```python
from build123d import *
from build123d import SkipClean  # not in build123d's __all__

# Parameters (mm, degrees)
F0_R     = 2.032
F1_DEPTH = 4.7625
F2_W     = 10.16
F2_H     = 58.42
F3_DEPTH = 6.35


with BuildPart() as f1:
    # F0 (on Top) → F1 (new body, symmetric)
    with BuildSketch(Plane.XY):
        with BuildLine():
            Line((0, -37.2616276145), (0, -45.72))
            add(Edge.make_bspline(
                [(0, -45.72), (28.8508510644, -45.72), (44.8791016558, -25.4)],
                knots=[1.5707963268, 1.5707963268, 1.5707963268, 2.5525616834, 2.5525616834, 2.5525616834], degree=2, weights=[1, 0.8819171037, 1]))
            Line((44.8791016558, -25.4), (44.8791016558, -23.9395))
            Line((44.8791016558, -23.9395), (37.2591016558, -23.9395))
            Line((37.2591016558, -23.9395), (37.2591016558, -19.4183))
            Line((37.2591016558, -19.4183), (30.7821016558, -19.4183))
            Line((30.7821016558, -19.4183), (30.7821016558, -21.1963))
            Line((30.7821016558, -21.1963), (26.7181016558, -21.1963))
            Line((26.7181016558, -21.1963), (26.7181016558, -13.5763))
            Line((26.7181016558, -13.5763), (30.7821016558, -13.5763))
            Line((30.7821016558, -13.5763), (30.7821016558, -15.3543))
            Line((30.7821016558, -15.3543), (37.2591016558, -15.3543))
            Line((37.2591016558, -15.3543), (37.2591016558, 15.2273))
            Line((37.2591016558, 15.2273), (30.7821016558, 15.2273))
            Line((30.7821016558, 15.2273), (30.7821016558, 13.4493))
            Line((30.7821016558, 13.4493), (26.7181016558, 13.4493))
            Line((26.7181016558, 13.4493), (26.7181016558, 21.0693))
            Line((26.7181016558, 21.0693), (30.7821016558, 21.0693))
            Line((30.7821016558, 21.0693), (30.7821016558, 19.2913))
            Line((30.7821016558, 19.2913), (37.2591016558, 19.2913))
            Line((37.2591016558, 19.2913), (37.2591016558, 23.8125))
            Line((37.2591016558, 23.8125), (44.8791016558, 23.8125))
            Line((44.8791016558, 23.8125), (44.8791016558, 25.4))
            add(Edge.make_bspline(
                [(44.8791016558, 25.4), (28.8508510644, 45.72), (0, 45.72)],
                knots=[3.7306236238, 3.7306236238, 3.7306236238, 4.7123889804, 4.7123889804, 4.7123889804], degree=2, weights=[1, 0.8819171037, 1]))
            Line((0, 45.72), (0, 29.7815))
            ThreePointArc((0, 29.7815), (2.0955, 27.686), (0, 25.5905))
            Line((0, 25.5905), (0, 17.1200428158))
            Line((0, 17.1200428158), (1.3565140544, 17.1200428158))
            Line((1.3565140544, 17.1200428158), (1.3565140544, 10.6807))
            Line((1.3565140544, 10.6807), (10.0905383006, 10.6807))
            Line((10.0905383006, 10.6807), (10.0905383006, -29.9593))
            Line((10.0905383006, -29.9593), (1.3565140544, -29.9593))
            Line((1.3565140544, -29.9593), (1.3565140544, -37.2616276145))
            Line((1.3565140544, -37.2616276145), (0, -37.2616276145))
        make_face()
        with Locations((5.0038, -33.7566)):
            Circle(F0_R, mode=Mode.SUBTRACT)
        with Locations((16.764, -22.225)):
            Circle(F0_R, mode=Mode.SUBTRACT)
        with Locations((5.0038, 14.478)):
            Circle(F0_R, mode=Mode.SUBTRACT)
    extrude(amount=F1_DEPTH, both=True)

    # F2 (on face) → F3 (cut)
    with BuildSketch(Plane.XY.offset(4.7625)):
        with Locations((5.08, -9.8651262736)):
            Rectangle(F2_W, F2_H)
    extrude(amount=-F3_DEPTH, mode=Mode.SUBTRACT)

    # F4: F1 across plane


with BuildPart() as f1_1:
    add(f1.part, clean=False)
    with SkipClean():  # cleaning this boolean's faces spoils the solid; the shape is the same uncleaned
        add(f1.part.mirror(Plane.YZ), clean=False)


solid = f1_1.part
```
The listing builds one solid part. Answer for the finished solid, in the listing's coordinates (mm). A direction names the side the tool comes from. Coordinates: 2 decimals unless noted, no trailing zeros. Write each loop counter-clockwise with the first axis right and the second up, starting at its lowest first coordinate (ties: lowest second). Pieces come first, ordered by that corner, then holes. Notation, with made-up numbers: (-7, -21.75) - (32, -21.75) arc R33 ccw to (32, 7.25) - close; hole circle Ø7 at (21.5, 46). An arc over 180 degrees is marked (long way). One line per item, written item: value.
1) Find section B-B (x = 34). Count the separate pieces of the cut face and the enclosed holes in it, and give its area (3 significant figures).
Geometry check:
separate pieces: 3
enclosed holes: 0
area: 599 mm2
2) For a pull along X with two mould halves and no side action, classify faces 5 (the flat face through (-37.259, -22, 0)), 6 (the flat face through (0, -37.262, -3)), 7 (the flat face through (34, 19.291, 0)) as pulls with the +X half, pulls with the -X half, needs draft (parallel to the pull), parting line crosses it, or undercut.
Geometry check:
face 5: pulls with the -X half
face 6: undercut
face 7: needs draft
3) Each of these flat-tipped pins is pushed along its axis until it touches: pin 1 Ø1 at (x, z) = (-35.5, 1) entering from -Y; pin 2 Ø1 at (x, z) = (-7.5, -3.5) entering from -Y; pin 3 Ø2.5 at (y, z) = (18.5, 0.5) entering from +X; pin 4 Ø3.5 at (x, y) = (16.764, -22.225) entering from -Z. Where does it stop, or does it pass through?
Geometry check:
pin 1: stops at y = -34.8
pin 2: stops at y = -45.33
pin 3: stops at x = 37.26
pin 4: passes through
4) Consider line 1 along Y through (x, z) = (0, 3); line 2 along X through (y, z) = (17, -3.75); line 3 along X through (y, z) = (-19, 0.25). Determine where each line is inside the solid, lowest interval first. Write a range as from..to.
Geometry check:
line 1: y = -45.72..-39.08, 19.34..25.59, 29.78..45.72
line 2: x = -26.72..-1.36, 1.36..26.72
line 3: x = -26.72..-10.16, 10.16..26.72
5) Find section A-A (y = 1.5). Give the vertices of the cut face in (x, z).
Geometry check:
outline: (-37.26, -4.76) - (-10.09, -4.76) - (-10.09, -1.59) - (-10.16, -1.59) - (-10.16, 4.76) - (-37.26, 4.76) - close; (10.09, -4.76) - (37.26, -4.76) - (37.26, 4.76) - (10.16, 4.76) - (10.16, -1.59) - (10.09, -1.59) - close
6) A tool of negligible diameter and unlimited length cuts with its end or side. For faces 1 (the flat face through (29, -13.576, 0)), 2 (the flat face through (34, -15.354, 0)), 3 (the flat face through (10.16, -10, 2)), 4 (the flat face through (-34, 19.291, 0)), from which of +Z, -Z, +X, -X, +Y, -Y can it reach the whole face along a straight path? Write none if from no direction.
Geometry check:
face 1: +Z, -Z
face 2: +Z, -Z, +X
face 3: +Z
face 4: +Z, -Z, -X
